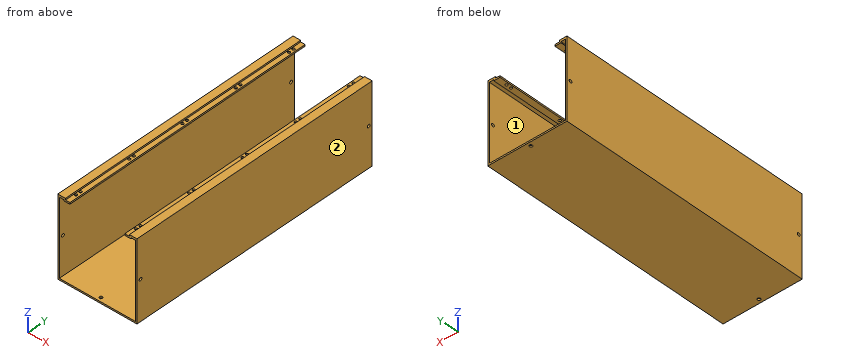
```python
from build123d import *

# Parameters (mm, degrees)
BOSS_EXTRUDE1_DEPTH = 327.5
SKETCH2_R           = 1.6
CUT_EXTRUDE2_DEPTH  = 10
SKETCH3_R           = 1.93
CUT_EXTRUDE3_DEPTH  = 102
SKETCH4_R           = 1.93
CUT_EXTRUDE4_DEPTH  = 10


with BuildPart() as part:
    # Sketch1 → Boss-Extrude1 (new body)
    with BuildSketch(Plane(origin=(0, 0, 0), x_dir=(1, 0, 0), z_dir=(0, 1, 0))):
        Polygon((0, -0.603), (0, 101.206), (101.206, 101.206), (101.206, -0.6), (91.5, -0.6), (91.5, 1.4), (85.703, 1.4), (85.703, 3.4), (93.5, 3.4), (93.5, 2), (99.206, 2), (99.206, 99.206), (2, 99.206), (2, 2), (7.706, 2), (7.706, 3.397), (15.503, 3.397), (15.503, 1.397), (9.706, 1.397), (9.706, -0.603), align=None)
    extrude(amount=BOSS_EXTRUDE1_DEPTH)

    # Sketch2 → Cut-Extrude2 (cut)
    with BuildSketch(Plane.XY.offset(-1.397)):
        with Locations((12.303, 314.9)):
            Circle(SKETCH2_R)
        with Locations((12.303, 308.5)):
            Circle(SKETCH2_R)
        with Locations((88.903, 314.9)):
            Circle(SKETCH2_R)
        with Locations((88.903, 308.5)):
            Circle(SKETCH2_R)
        with Locations((12.15225, 240.925)):
            Circle(SKETCH2_R)
        with Locations((12.15225, 234.525)):
            Circle(SKETCH2_R)
        with Locations((88.75225, 240.925)):
            Circle(SKETCH2_R)
        with Locations((88.75225, 234.525)):
            Circle(SKETCH2_R)
        with Locations((12.0015, 166.95)):
            Circle(SKETCH2_R)
        with Locations((12.0015, 160.55)):
            Circle(SKETCH2_R)
        with Locations((88.6015, 166.95)):
            Circle(SKETCH2_R)
        with Locations((88.6015, 160.55)):
            Circle(SKETCH2_R)
        with Locations((11.85075, 92.975)):
            Circle(SKETCH2_R)
        with Locations((11.85075, 86.575)):
            Circle(SKETCH2_R)
        with Locations((88.45075, 92.975)):
            Circle(SKETCH2_R)
        with Locations((88.45075, 86.575)):
            Circle(SKETCH2_R)
        with Locations((11.7, 19)):
            Circle(SKETCH2_R)
        with Locations((11.7, 12.6)):
            Circle(SKETCH2_R)
        with Locations((88.3, 19)):
            Circle(SKETCH2_R)
        with Locations((88.3, 12.6)):
            Circle(SKETCH2_R)
    extrude(amount=-CUT_EXTRUDE2_DEPTH, mode=Mode.SUBTRACT)

    # Sketch3 → Cut-Extrude3 (cut)
    with BuildSketch(Plane(origin=(101.206, 0, 0), x_dir=(0, 0, -1), z_dir=(1, 0, 0))):
        with Locations((50.603, 322.524)):
            Circle(SKETCH3_R)
        with Locations((50.603, 4.976)):
            Circle(SKETCH3_R)
    extrude(amount=-CUT_EXTRUDE3_DEPTH, mode=Mode.SUBTRACT)

    # Sketch4 → Cut-Extrude4 (cut)
    with BuildSketch(Plane(origin=(0, 0, -101.206), x_dir=(-1, 0, 0), z_dir=(0, 0, -1))):
        with Locations((-50.603, 322.524)):
            Circle(SKETCH4_R)
        with Locations((-50.603, 4.976)):
            Circle(SKETCH4_R)
    extrude(amount=-CUT_EXTRUDE4_DEPTH, mode=Mode.SUBTRACT)


solid = part.part
```
Design review of the part built by this model. Coordinates are the model's own, in mm. Face numbers are marked on the shaded views. A direction names the side the tool comes from. Round coordinates to 2 decimals unless told otherwise and drop trailing zeros. Write each loop counter-clockwise with the first axis right and the second up, starting at its lowest first coordinate (ties: lowest second). Pieces come first, ordered by that corner, then holes. Notation, with made-up numbers: (16, 68.25) -> (63, 68.25) arc R22 cw to (63, 79.25) -> close; hole circle Ø3 at (77.5, 60). An arc over 180 degrees is marked (long way). Write item = value, one per line. Start each with the question number.
1) Tool access review of the marked faces 1 and 2: name each direction out of +Z, -Z, +X, -X, +Y, -Y from which nothing blocks a thin tool from reaching the whole face with its end or side.
2) Wall thickness on probe 1 along X at (y, z) = (97, -30); probe 2 along Z at (x, y) = (94, 76); probe 3 along Z at (x, y) = (12, 70.5): over which ranges is each line inside the solid? List them lowest first. Write a range as from..to.
3) Clearance check with flat-ended pins moving along their axes: pin 1 (2.5 mm diameter, centred on x = 88.75, y = 240.92, fed in from +Z); pin 2 (4 mm diameter, centred on x = 88.45, y = 86.58, fed in from +Z); pin 3 (2.5 mm diameter, centred on y = 4.976, z = -50.603, fed in from +X). State where each tip first meets the part, or that it passes through.
4) Take a section at A-A, the plane z = -60. State the section outline as (x, y) points, plus the area to 3 significant figures.
5) Take a section at B-B, the plane y = 50.5. State the section outline as (x, z) points.
6) Take a section at C-C, the plane x = 65. State the section outline as (y, z) points, plus the area to 3 significant figures.
Results list:
q1.face_1 = +Y, -Y
q1.face_2 = +Z, -Z, +X, +Y, -Y
q2.probe_1 = 0..2, 99.21..101.21
q2.probe_2 = -101.21..-99.21, -2..0.6
q2.probe_3 = -101.21..-99.21, -3.4..-1.4
q3.pin_1 = -99.21
q3.pin_2 = -1.4
q3.pin_3 = through
q4.outline = (0, 0) -> (2, 0) -> (2, 327.5) -> (0, 327.5) -> close; (99.21, 0) -> (101.21, 0) -> (101.21, 327.5) -> (99.21, 327.5) -> close
q4.area = 1,310 mm²
q5.outline = (0, -101.21) -> (101.21, -101.21) -> (101.21, 0.6) -> (91.5, 0.6) -> (91.5, -1.4) -> (85.7, -1.4) -> (85.7, -3.4) -> (93.5, -3.4) -> (93.5, -2) -> (99.21, -2) -> (99.21, -99.21) -> (2, -99.21) -> (2, -2) -> (7.71, -2) -> (7.71, -3.4) -> (15.5, -3.4) -> (15.5, -1.4) -> (9.71, -1.4) -> (9.71, 0.6) -> (0, 0.6) -> close
q6.outline = (0, -101.21) -> (327.5, -101.21) -> (327.5, -99.21) -> (0, -99.21) -> close
q6.area = 655 mm²
